```python
from build123d import *

# Parameters (mm, degrees)
SKETCH1_W            = 25.5
SKETCH1_H            = 14
BOSS_EXTRUDE1_DEPTH  = 4
SKETCH2_R            = 1.5
CUT_EXTRUDE1_DEPTH   = 53.71750714
SKETCH3_W            = 30.5
SKETCH3_H            = 4
BOSS_EXTRUDE2_DEPTH  = 5.1
SKETCH4_W            = 30.5
SKETCH4_H            = 3
BOSS_EXTRUDE3_DEPTH  = 24
SKETCH5_W            = 30.5
SKETCH5_H            = 2
BOSS_EXTRUDE8_DEPTH  = 14.8
SKETCH10_W           = 30.5
SKETCH10_H           = 2
BOSS_EXTRUDE9_DEPTH  = 16.8
SKETCH11_W           = 1.5
SKETCH11_H           = 12.8
BOSS_EXTRUDE10_DEPTH = 4.6
SKETCH13_W           = 15.25
SKETCH13_H           = 2
BOSS_EXTRUDE11_DEPTH = 15.75
SKETCH14_W           = 10
SKETCH14_H           = 5
CUT_EXTRUDE5_DEPTH   = 3
SKETCH16_R           = 1
CUT_EXTRUDE6_DEPTH   = 10
SKETCH15_W           = 14.75
SKETCH15_H           = 3
BOSS_EXTRUDE12_DEPTH = 6.55


with BuildPart() as part:
    # Sketch1 → Boss-Extrude1 (new body)
    with BuildSketch(Plane(origin=(0, 0, 0), x_dir=(1, 0, 0), z_dir=(0, 1, 0))):
        Polygon((-36.234375, 20.8984375), (-41.234375, 20.8984375), (-41.234375, -32.6015625), (-36.234375, -32.6015625), (-36.234375, 6.8984375), align=None)
        with Locations((-23.484375, 13.8984375)):
            Rectangle(SKETCH1_W, SKETCH1_H)
    extrude(amount=BOSS_EXTRUDE1_DEPTH)

    # Sketch2 → Cut-Extrude1 (cut, through all)
    with BuildSketch(Plane(origin=(0, 4, 0), x_dir=(1, 0, 0), z_dir=(0, 1, 0))):
        with Locations(Location((-38.984375, -29.3515625, 0), (0, 0, 270))):
            Circle(SKETCH2_R)
        with Locations(Location((-38.984375, 12.6484375, 0), (0, 0, 270))):
            Circle(SKETCH2_R)
        with Locations(Location((-13.984375, 12.6484375, 0), (0, 0, 270))):
            Circle(SKETCH2_R)
    extrude(amount=-CUT_EXTRUDE1_DEPTH, mode=Mode.SUBTRACT)

    # Sketch3 → Boss-Extrude2 (add)
    with BuildSketch(Plane(origin=(0, 0, -20.8984375), x_dir=(-1, 0, 0), z_dir=(0, 0, -1))):
        with Locations((25.984375, 2)):
            Rectangle(SKETCH3_W, SKETCH3_H)
    extrude(amount=BOSS_EXTRUDE2_DEPTH)

    # Sketch4 → Boss-Extrude3 (add)
    with BuildSketch(Plane.XZ):
        with Locations((-25.984375, -24.4984375)):
            Rectangle(SKETCH4_W, SKETCH4_H)
    extrude(amount=BOSS_EXTRUDE3_DEPTH)

    # Sketch5 → Boss-Extrude8 (add)
    with BuildSketch(Plane(origin=(0, 0, -25.9984375), x_dir=(-1, 0, 0), z_dir=(0, 0, -1))):
        with Locations((25.984375, -23)):
            Rectangle(SKETCH5_W, SKETCH5_H)
    extrude(amount=BOSS_EXTRUDE8_DEPTH)

    # Sketch10 → Boss-Extrude9 (add)
    with BuildSketch(Plane(origin=(0, -22, 0), x_dir=(1, 0, 0), z_dir=(0, 1, 0))):
        with Locations((-25.984375, 39.7984375)):
            Rectangle(SKETCH10_W, SKETCH10_H)
    extrude(amount=BOSS_EXTRUDE9_DEPTH)

    # Sketch11 → Boss-Extrude10 (add)
    with BuildSketch(Plane(origin=(0, -22, 0), x_dir=(1, 0, 0), z_dir=(0, 1, 0))):
        with Locations((-11.484375, 32.3984375)):
            Rectangle(SKETCH11_W, SKETCH11_H)
    boss_extrude10 = extrude(amount=BOSS_EXTRUDE10_DEPTH)

    # Sketch13 → Boss-Extrude11 (add)
    with BuildSketch(Plane(origin=(0, -5.2, 0), x_dir=(1, 0, 0), z_dir=(0, 1, 0))):
        with Locations((-18.359375, 39.7984375)):
            Rectangle(SKETCH13_W, SKETCH13_H)
    extrude(amount=BOSS_EXTRUDE11_DEPTH)

    # Sketch14 → Cut-Extrude5 (cut)
    with BuildSketch(Plane.XY.offset(-22.9984375)):
        with Locations((-30.706752917, -18.5)):
            Rectangle(SKETCH14_W, SKETCH14_H)
    extrude(amount=-CUT_EXTRUDE5_DEPTH, mode=Mode.SUBTRACT)

    # Sketch16 → Cut-Extrude6 (cut)
    with BuildSketch(Plane(origin=(-10.734375, 0, 0), x_dir=(0, 0, -1), z_dir=(1, 0, 0))):
        with Locations((32.3984375, -19.4)):
            Circle(SKETCH16_R)
    cut_extrude6 = extrude(amount=-CUT_EXTRUDE6_DEPTH, mode=Mode.SUBTRACT)

    # Mirror1: Boss-Extrude10, Cut-Extrude6 across plane
    add(boss_extrude10.mirror(Plane(origin=(0, -5.725, 0), x_dir=(0, 0, 1), z_dir=(0, -1, 0))))
    add(cut_extrude6.mirror(Plane(origin=(0, -5.725, 0), x_dir=(0, 0, 1), z_dir=(0, -1, 0))), mode=Mode.SUBTRACT)

    # Sketch15 → Boss-Extrude12 (add)
    with BuildSketch(Plane(origin=(0, 4, 0), x_dir=(1, 0, 0), z_dir=(0, 1, 0))):
        with Locations((-18.109375, 24.4984375)):
            Rectangle(SKETCH15_W, SKETCH15_H)
    extrude(amount=BOSS_EXTRUDE12_DEPTH)


solid = part.part
```
Geometry check sheet. Reference: the model listing, model coordinates, mm. A direction names the side the tool comes from. Coordinates: 2 decimals unless noted, no trailing zeros. Order: outer loops, then holes, each group sorted by start corner. A loop starts at its lowest first (then second) coordinate and runs counter-clockwise, first axis right, second up.
Item 1: Depth check by flat-ended pin: pin 1 (1.8 mm diameter, centred on y = 7.95, z = -32.4, fed in from -X); pin 2 (1.5 mm diameter, centred on x = -29.5, y = -18, fed in from +Z); pin 3 (2 mm diameter, centred on x = -17.5, y = 2, fed in from +Z); pin 4 (2 mm diameter, centred on x = -17, y = 7, fed in from +Z). Enter the tip coordinate at first touch or a pass-through.
Item 2: Tool access check on faces 5 (the flat face through (-34, -5.2, -40)), 6 (the flat face through (-18, 7, -22.998)), 7 (the flat face through (-26, -12, -22.998)), 8 (the flat face through (-27, -22, -32)), 9 (the flat face through (-31, -16, -24)). Record the directions out of +Z, -Z, +X, -X, +Y, -Y that give a thin tool (end or side, any length) a straight path to the whole face; none if there is none.
Item 3: Scan lines: line 1 along Z through (x, y) = (-16.5, -19); line 2 along Z through (x, y) = (-23, 3); line 3 along Z through (x, y) = (-40, -2). Record each from-to range of solid material in increasing order.
Item 4: Section check D-D (z = -12). Enter the section's corners in (x, y), plus the area to 3 significant figures.
Item 5: Section check C-C (y = -19.4). Enter the section's corners in (x, z), plus the area to 3 significant figures.
Item 6: Section check A-A (y = -4.5). Enter the section's corners in (x, z), plus the area to 3 significant figures.
Item 7: Section check B-B (x = -34.5). Enter the section's corners in (y, z).
Item 8: Mould release check, pull along Y, two halves, no side actions. Record for faces 1 (the flat face through (-29.2, 0, -7.2)), 2 (the flat face through (-23, -11, -40.798)), 3 (the flat face through (-35.707, -19, -24)), 4 (the cylindrical face through (-11.5, 7.9, -31.4)): released by +Y, released by -Y, zero draft, split by the parting line, or undercut.
Check sheet entries:
1. pin 1: passes through
1. pin 2: stops at z = -38.8
1. pin 3: stops at z = -6.9
1. pin 4: stops at z = -23
2. face 5: -Z, -X, +Y
2. face 6: +Z, +X, -X, +Y
2. face 7: +Z, +X, -X, -Y
2. face 8: -X, +Y
2. face 9: +Z
3. line 1: z = -40.8 to -38.8, -26 to -23
3. line 2: z = -40.8 to -38.8, -26 to -6.9
3. line 3: z = -26 to -23
4. outline: (-41.23, 0) - (-40.34, 0) - (-40.34, 4) - (-41.23, 4) - close; (-37.63, 0) - (-15.34, 0) - (-15.34, 4) - (-37.63, 4) - close; (-12.63, 0) - (-10.73, 0) - (-10.73, 4) - (-12.63, 4) - close
4. area: 100 mm2
5. outline: (-41.23, -40.8) - (-10.73, -40.8) - (-10.73, -33.4) - (-12.23, -33.4) - (-12.23, -38.8) - (-41.23, -38.8) - close; (-41.23, -26) - (-35.71, -26) - (-35.71, -23) - (-41.23, -23) - close; (-25.71, -26) - (-12.23, -26) - (-12.23, -31.4) - (-10.73, -31.4) - (-10.73, -23) - (-25.71, -23) - close
5. area: 139 mm2
6. outline: (-41.23, -26) - (-10.73, -26) - (-10.73, -23) - (-41.23, -23) - close; (-25.98, -40.8) - (-10.73, -40.8) - (-10.73, -38.8) - (-25.98, -38.8) - close
6. area: 122 mm2
7. outline: (-24, -40.8) - (-5.2, -40.8) - (-5.2, -38.8) - (-22, -38.8) - (-22, -26) - (-21, -26) - (-21, -23) - (-24, -23) - close; (-16, -26) - (4, -26) - (4, -6.9) - (0, -6.9) - (0, -23) - (-16, -23) - close
8. face 1: released by -Y
8. face 2: zero draft
8. face 3: undercut
8. face 4: undercut
